from build123d import *

# Parameters (mm, degrees)
PLACA_START                     = 4
PLACA_DEPTH                     = 6.35
PLACA_R1_START                  = 4
CROQUIS14_R                     = 35
PLACA_R1_DEPTH                  = 6.35
PLACA_R2_START                  = 4
CROQUIS15_R                     = 30
PLACA_R2_DEPTH                  = 6.35
ALIGERADO_START                 = 4
ALIGERADO_DEPTH                 = 6.35
BARRENOS_SEPARADORES_M4_START   = 4
CROQUIS17_R                     = 2.25
BARRENOS_SEPARADORES_M4_DEPTH   = 6.35
BARRENOS_M2_Y_M3_START          = 4
CROQUIS18_R                     = 2.25
CROQUIS18_R_2                   = 2.6
CROQUIS18_R_3                   = 5.5
CROQUIS18_R_4                   = 18
CROQUIS18_R_5                   = 1.45
BARRENOS_M2_Y_M3_DEPTH          = 6.35
REFRENTADO_M4_CABEZA_BAJA_START = 4
CROQUIS19_R                     = 4
REFRENTADO_M4_CABEZA_BAJA_DEPTH = 2.8
REFRENTADO_M2_5_START           = 4
CROQUIS20_R                     = 2.8
REFRENTADO_M2_5_DEPTH           = 2.6
ROSCA_M3_BASES_CINCHO_START     = 4
CROQUIS21_R                     = 1.25
ROSCA_M3_BASES_CINCHO_DEPTH     = 6.35
PASO_M3_BASES_CINCHO_START      = 4
CROQUIS22_R                     = 1.7
PASO_M3_BASES_CINCHO_DEPTH      = 6.35


with BuildPart() as part:
    # Croquis13 → Placa (new body)
    with BuildSketch(Plane(origin=(0, 0, 0), x_dir=(1, 0, 0), z_dir=(0, 1, 0)).offset(PLACA_START)):
        Polygon((1.148293963, -206.431158085), (153.384251969, -201.433849787), (153.384251969, -141.466150213), (1.148293963, -136.468841915), align=None)
    extrude(amount=PLACA_DEPTH)

    # Croquis14 → Placa_r1 (add)
    with BuildSketch(Plane(origin=(0, 0, 0), x_dir=(1, 0, 0), z_dir=(0, 1, 0)).offset(PLACA_R1_START)):
        with Locations((0, -171.45)):
            Circle(CROQUIS14_R)
    extrude(amount=PLACA_R1_DEPTH)

    # Croquis15 → Placa_r2 (add)
    with BuildSketch(Plane(origin=(0, 0, 0), x_dir=(1, 0, 0), z_dir=(0, 1, 0)).offset(PLACA_R2_START)):
        with Locations((152.4, -171.45)):
            Circle(CROQUIS15_R)
    extrude(amount=PLACA_R2_DEPTH)

    # Croquis16 → Aligerado (cut)
    with BuildSketch(Plane(origin=(0, 0, 0), x_dir=(1, 0, 0), z_dir=(0, 1, 0)).offset(ALIGERADO_START)):
        with BuildLine():
            Line((55, -162.45), (75, -162.45))
            ThreePointArc((75, -162.45), (84, -171.45), (75, -180.45))
            Line((75, -180.45), (55, -180.45))
            ThreePointArc((55, -180.45), (46, -171.45), (55, -162.45))
        make_face()
    extrude(amount=ALIGERADO_DEPTH, mode=Mode.SUBTRACT)

    # Croquis17 → Barrenos_separadores_M4 (cut)
    with BuildSketch(Plane(origin=(0, 0, 0), x_dir=(1, 0, 0), z_dir=(0, 1, 0)).offset(BARRENOS_SEPARADORES_M4_START)):
        with Locations(Location((40, -195.45, 0), (0, 0, 270))):
            Circle(CROQUIS17_R)
        with Locations(Location((40, -147.45, 0), (0, 0, 270))):
            Circle(CROQUIS17_R)
        with Locations(Location((90, -191.45, 0), (0, 0, 270))):
            Circle(CROQUIS17_R)
        with Locations(Location((90, -151.45, 0), (0, 0, 270))):
            Circle(CROQUIS17_R)
    extrude(amount=BARRENOS_SEPARADORES_M4_DEPTH, mode=Mode.SUBTRACT)

    # Croquis18 → Barrenos_M2_y_M3 (cut)
    with BuildSketch(Plane(origin=(0, 0, 0), x_dir=(1, 0, 0), z_dir=(0, 1, 0)).offset(BARRENOS_M2_Y_M3_START)):
        with Locations(Location((12.990381057, -178.95, 0), (0, 0, 270))):
            Circle(CROQUIS18_R)
        with Locations(Location((0, -186.45, 0), (0, 0, 270))):
            Circle(CROQUIS18_R)
        with Locations(Location((-12.990381057, -178.95, 0), (0, 0, 270))):
            Circle(CROQUIS18_R)
        with Locations(Location((-12.990381057, -163.95, 0), (0, 0, 270))):
            Circle(CROQUIS18_R)
        with Locations(Location((0, -156.45, 0), (0, 0, 270))):
            Circle(CROQUIS18_R)
        with Locations(Location((12.990381057, -163.95, 0), (0, 0, 270))):
            Circle(CROQUIS18_R)
        with Locations(Location((7.125, -183.790862004, 0), (0, 0, 270))):
            Circle(CROQUIS18_R_2)
        with Locations(Location((-14.25, -171.45, 0), (0, 0, 270))):
            Circle(CROQUIS18_R_2)
        with Locations(Location((7.125, -159.109137996, 0), (0, 0, 270))):
            Circle(CROQUIS18_R_2)
        with Locations(Location((0, -171.45, 0), (0, 0, 270))):
            Circle(CROQUIS18_R_3)
        with Locations(Location((152.4, -171.45, 0), (0, 0, 270))):
            Circle(CROQUIS18_R_4)
        with Locations(Location((172.65, -171.45, 0), (0, 0, 270))):
            Circle(CROQUIS18_R_5)
        with Locations(Location((166.718912319, -185.768912319, 0), (0, 0, 270))):
            Circle(CROQUIS18_R_5)
        with Locations(Location((152.4, -191.7, 0), (0, 0, 270))):
            Circle(CROQUIS18_R_5)
        with Locations(Location((138.081087681, -185.768912319, 0), (0, 0, 270))):
            Circle(CROQUIS18_R_5)
        with Locations(Location((132.15, -171.45, 0), (0, 0, 270))):
            Circle(CROQUIS18_R_5)
        with Locations(Location((138.081087681, -157.131087681, 0), (0, 0, 270))):
            Circle(CROQUIS18_R_5)
        with Locations(Location((152.4, -151.2, 0), (0, 0, 270))):
            Circle(CROQUIS18_R_5)
        with Locations(Location((166.718912319, -157.131087681, 0), (0, 0, 270))):
            Circle(CROQUIS18_R_5)
    extrude(amount=BARRENOS_M2_Y_M3_DEPTH, mode=Mode.SUBTRACT)

    # Croquis19 → Refrentado_M4_cabeza_baja (cut)
    with BuildSketch(Plane(origin=(0, 0, 0), x_dir=(1, 0, 0), z_dir=(0, 1, 0)).offset(REFRENTADO_M4_CABEZA_BAJA_START)):
        with Locations(Location((12.990381057, -178.95, 0), (0, 0, 270))):
            Circle(CROQUIS19_R)
        with Locations(Location((0, -186.45, 0), (0, 0, 270))):
            Circle(CROQUIS19_R)
        with Locations(Location((-12.990381057, -178.95, 0), (0, 0, 270))):
            Circle(CROQUIS19_R)
        with Locations(Location((-12.990381057, -163.95, 0), (0, 0, 270))):
            Circle(CROQUIS19_R)
        with Locations(Location((0, -156.45, 0), (0, 0, 270))):
            Circle(CROQUIS19_R)
        with Locations(Location((12.990381057, -163.95, 0), (0, 0, 270))):
            Circle(CROQUIS19_R)
    extrude(amount=REFRENTADO_M4_CABEZA_BAJA_DEPTH, mode=Mode.SUBTRACT)

    # Croquis20 → Refrentado_M2-5 (cut)
    with BuildSketch(Plane(origin=(0, 0, 0), x_dir=(1, 0, 0), z_dir=(0, 1, 0)).offset(REFRENTADO_M2_5_START)):
        with Locations((172.65, -171.45)):
            Circle(CROQUIS20_R)
        with Locations((166.718912319, -185.768912319)):
            Circle(CROQUIS20_R)
        with Locations((152.4, -191.7)):
            Circle(CROQUIS20_R)
        with Locations((138.081087681, -185.768912319)):
            Circle(CROQUIS20_R)
        with Locations((132.15, -171.45)):
            Circle(CROQUIS20_R)
        with Locations((138.081087681, -157.131087681)):
            Circle(CROQUIS20_R)
        with Locations((152.4, -151.2)):
            Circle(CROQUIS20_R)
        with Locations((166.718912319, -157.131087681)):
            Circle(CROQUIS20_R)
    extrude(amount=REFRENTADO_M2_5_DEPTH, mode=Mode.SUBTRACT)

    # Croquis21 → Rosca_M3_bases_cincho (cut)
    with BuildSketch(Plane(origin=(0, 0, 0), x_dir=(1, 0, 0), z_dir=(0, 1, 0)).offset(ROSCA_M3_BASES_CINCHO_START)):
        with Locations(Location((112, -171.45, 0), (0, 0, 270))):
            Circle(CROQUIS21_R)
    extrude(amount=ROSCA_M3_BASES_CINCHO_DEPTH, mode=Mode.SUBTRACT)

    # Croquis22 → Paso_M3_bases_cincho (cut)
    with BuildSketch(Plane(origin=(0, 0, 0), x_dir=(1, 0, 0), z_dir=(0, 1, 0)).offset(PASO_M3_BASES_CINCHO_START)):
        with Locations(Location((112, -171.45, 0), (0, 0, 270))):
            Circle(CROQUIS22_R)
    extrude(amount=PASO_M3_BASES_CINCHO_DEPTH, mode=Mode.SUBTRACT)


solid = part.part
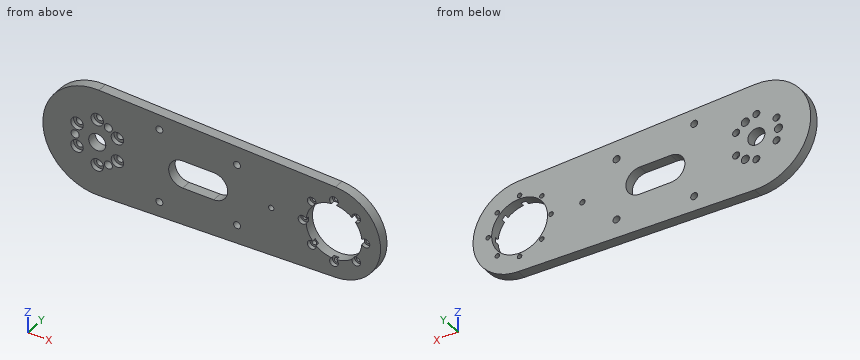
The model under review builds one solid part; all positions refer to its coordinate system, in mm. Give positions to 0.01 mm unless a question says otherwise; leave off trailing zeros. Order: outer loops, then holes, each group sorted by start corner. A loop starts at its lowest first (then second) coordinate and runs counter-clockwise, first axis right, second up. Notation, with made-up numbers: M 24,-32 L 58,-32 A16 ccw 58,-27 Z; hole C 88.25,20.5 d11. An arc over 180 degrees is marked long. Use one line per item in the form item = value. Start each with the question number.
Item 1: We need section B-B on y = 8.75. Give the number of separate pieces and of enclosed holes in the cut face, plus the area to 3 significant figures.
Item 2: To check wall thickness, follow line 1 along X through (y, z) = (5, 171.45); line 2 along X through (y, z) = (8.75, 157); line 3 along X through (y, z) = (8.75, 175). State the ranges of each line that lie inside material, in increasing order. Write a range as from..to.
Item 3: We need section A-A on x = 66. Give the boundary of the cut face in (y, z), plus the area to 3 significant figures.
Item 4: Insertion check: pin 1 Ø1.5 at (x, z) = (151.5, 151) entering from -Y; pin 2 Ø1 at (x, y) = (99.5, 9) entering from -Z; pin 3 Ø7 at (x, z) = (12.99, 163.95) entering from -Y. Each pin has a flat end and moves straight along its axis. Give the tip position at first contact, or say it passes through.
Completed:
q1.separate_pieces = 1
q1.enclosed_holes = 25
q1.area = 11,200 mm²
q2.line_1 = -35..-16.85, -11.65..-5.5, 5.5..46, 84..110.3, 113.7..129.35, 175.45..182.4
q2.line_2 = -31.88..-2.18, 2.18..5.6, 8.65..136.64, 139.53..141.67, 163.13..165.27, 168.16..178.69
q2.line_3 = -34.82..-4.2, 4.2..46.73, 83.27..134.75, 170.05..182.19
q3.outline = M 4,138.6 L 10.35,138.6 L 10.35,162.45 L 4,162.45 Z; M 4,180.45 L 10.35,180.45 L 10.35,204.3 L 4,204.3 Z
q3.area = 303 mm²
q4.pin_1 = 6.6
q4.pin_2 = 139.68
q4.pin_3 = 6.8
